For this review, take the finished solid that the model builds, in its own axes (mm). Face numbers are marked on the shaded views. A direction names the side the tool comes from. Coordinates: 2 decimals unless noted, no trailing zeros. Loops run counter-clockwise (first coordinate to the right, second up) from the corner with the lowest first, then second, coordinate; pieces in that order, holes last. Notation, with made-up numbers: M 88.5,-40 L 119.5,-40 A21 ccw 119.5,-11 Z; hole C 31,57 d10. An arc over 180 degrees is marked long. Put each result on its own line as item: value.
```python
from build123d import *

# Parameters (mm, degrees)
SKETCH1_W           = 60
SKETCH1_H           = 50
BOSS_EXTRUDE1_DEPTH = 12
SKETCH2_R           = 11
CUT_EXTRUDE1_DEPTH  = 2
CUT_EXTRUDE2_REACH  = 42.853
SKETCH3_R           = 5
CUT_EXTRUDE3_REACH  = 61.532
SKETCH4_R           = 3
CUT_EXTRUDE5_REACH  = 42.311
SKETCH6_R           = 12


with BuildPart() as part:
    # Sketch1 → Boss-Extrude1 (new body)
    with BuildSketch(Plane.XY):
        Rectangle(SKETCH1_W, SKETCH1_H)
    extrude(amount=BOSS_EXTRUDE1_DEPTH)

    # Sketch2 → Cut-Extrude1 (cut)
    with BuildSketch(Plane.XY.offset(12)):
        with Locations((0, 4.5)):
            Circle(SKETCH2_R)
    extrude(amount=-CUT_EXTRUDE1_DEPTH, mode=Mode.SUBTRACT)

    # Sketch3 → Cut-Extrude2 (cut, up to next)
    with BuildSketch(Plane.XY.offset(12), mode=Mode.PRIVATE) as cut_extrude2_sk1:
        with Locations((-20, -5)):
            Circle(SKETCH3_R)
    cut_extrude2_tool1 = extrude(cut_extrude2_sk1.sketch, amount=-CUT_EXTRUDE2_REACH, mode=Mode.PRIVATE) & part.part
    # Sketch3 → Cut-Extrude2 (cut, up to next)
    with BuildSketch(Plane.XY.offset(12), mode=Mode.PRIVATE) as cut_extrude2_sk2:
        with Locations((20, -5)):
            Circle(SKETCH3_R)
    cut_extrude2_tool2 = extrude(cut_extrude2_sk2.sketch, amount=-CUT_EXTRUDE2_REACH, mode=Mode.PRIVATE) & part.part
    add(cut_extrude2_tool1.solids().sort_by_distance((-20, -5, 12))[0], mode=Mode.SUBTRACT)
    add(cut_extrude2_tool2.solids().sort_by_distance((20, -5, 12))[0], mode=Mode.SUBTRACT)

    # Sketch4 → Cut-Extrude3 (cut, up to next)
    with BuildSketch(Plane.XZ.offset(25), mode=Mode.PRIVATE) as cut_extrude3_sk1:
        with Locations(Location((20, 6, 0), (0, 0, 270))):
            Circle(SKETCH4_R)
    cut_extrude3_tool1 = extrude(cut_extrude3_sk1.sketch, amount=-CUT_EXTRUDE3_REACH, mode=Mode.PRIVATE) & part.part
    # Sketch4 → Cut-Extrude3 (cut, up to next)
    with BuildSketch(Plane.XZ.offset(25), mode=Mode.PRIVATE) as cut_extrude3_sk2:
        with Locations(Location((-20, 6, 0), (0, 0, 270))):
            Circle(SKETCH4_R)
    cut_extrude3_tool2 = extrude(cut_extrude3_sk2.sketch, amount=-CUT_EXTRUDE3_REACH, mode=Mode.PRIVATE) & part.part
    add(cut_extrude3_tool1.solids().sort_by_distance((20, -25, 6))[0], mode=Mode.SUBTRACT)
    add(cut_extrude3_tool2.solids().sort_by_distance((-20, -25, 6))[0], mode=Mode.SUBTRACT)

    # Sketch6 → Cut-Extrude5 (cut, up to next)
    with BuildSketch(Plane.XY.offset(10), mode=Mode.PRIVATE) as cut_extrude5_sk1:
        with Locations((0, 4.5)):
            Circle(SKETCH6_R)
    cut_extrude5_tool1 = extrude(cut_extrude5_sk1.sketch, amount=-CUT_EXTRUDE5_REACH, mode=Mode.PRIVATE) & part.part
    add(cut_extrude5_tool1.solids().sort_by_distance((0, 4.5, 10))[0], mode=Mode.SUBTRACT)


solid = part.part
```
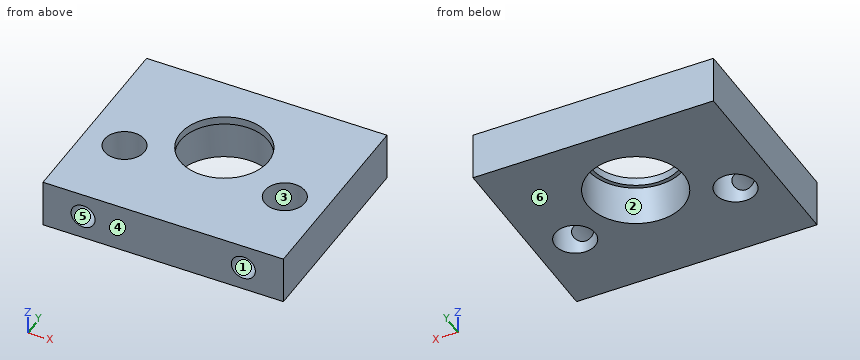
(1) Add section A-A (y = 4.5). Write out the cut boundary in (x, z).
Determined:
outline: M -30,0 L -12,0 L -12,10 L -11,10 L -11,12 L -30,12 Z; M 11,10 L 12,10 L 12,0 L 30,0 L 30,12 L 11,12 Z
(2) Add section D-D (y = -20). Write out the cut boundary in (x, z), plus the area to 3 significant figures.
Determined:
outline: M -30,0 L 30,0 L 30,12 L -30,12 Z; hole C -20,6 d6; hole C 20,6 d6
area: 663 mm^2
(3) For pin 1 (5.5 mm diameter, centred on x = 20, z = 6, fed in from -Y); pin 2 (3.5 mm diameter, centred on x = -20, z = 6, fed in from -Y), all flat-tipped, find the tip position at first contact; note any pin that passes through.
Determined:
pin 1: stops at y = -0.82
pin 2: stops at y = -0.32
(4) Draft analysis for pull direction Z (two halves, no side actions). For the marked faces 4, 5 and 6, state which applies: +Z half, -Z half, draft (parallel to the pull), parting line (faces both ways), or undercut.
Determined:
face 4: draft
face 5: undercut
face 6: -Z half
(5) Add section B-B (x = -1.5). Write out the cut boundary in (y, z).
Determined:
outline: M -25,0 L -7.41,0 L -7.41,10 L -6.4,10 L -6.4,12 L -25,12 Z; M 15.4,10 L 16.41,10 L 16.41,0 L 25,0 L 25,12 L 15.4,12 Z
(6) Tool access review of the marked faces 1, 2 and 3: name each direction out of +Z, -Z, +X, -X, +Y, -Y from which nothing blocks a thin tool from reaching the whole face with its end or side.
Determined:
face 1: -Y
face 2: -Z
face 3: +Z, -Z
(7) Add section C-C (z = 6). Write out the cut boundary in (x, y), plus the area to 3 significant figures.
Determined:
outline: M -30,-25 L -23,-25 L -23,-9 A5 cw long -17,-9 L -17,-25 L 17,-25 L 17,-9 A5 cw long 23,-9 L 23,-25 L 30,-25 L 30,25 L -30,25 Z; hole C 0,4.5 d24
area: 2,210 mm^2
(8) Wall thickness on line 1 along X through (y, z) = (-17, 6.25); line 2 along Z through (x, y) = (-20, -20); line 3 along Y through (x, z) = (20, 5.75): over which ranges is each line inside the solid? List them lowest first. Write a range as [from, to].
Determined:
line 1: x = [-30, -22.99], [-17.01, 17.01], [22.99, 30]
line 2: z = [0, 3], [9, 12]
line 3: y = [0, 25]
